Geometry check sheet. Reference: the model listing, model coordinates, mm. Give positions to 0.01 mm unless a question says otherwise; leave off trailing zeros. Write each loop counter-clockwise with the first axis right and the second up, starting at its lowest first coordinate (ties: lowest second). Pieces come first, ordered by that corner, then holes.
(1) Cross-section at C-C (z = 0.85). Record the boundary of the cut face in (x, y) (1 decimal), and give its area (3 significant figures).
(2) Cross-section at B-B (y = 733.5). Record the boundary of the cut face in (x, z) (3 decimals), and give its area (3 significant figures).
(3) Cross-section at D-D (y = 767.5). Record the boundary of the cut face in (x, z) (3 decimals), and give its area (3 significant figures).
(4) Cross-section at A-A (x = -59). Record the boundary of the cut face in (y, z) (3 decimals).
(5) Thickness scan on line 1 along Y through (x, z) = (-29, 2.6); line 2 along Y through (x, z) = (-38, 2.15); line 3 along Y through (x, z) = (-48, 0.6). Record the ranges inside material, lowest first.
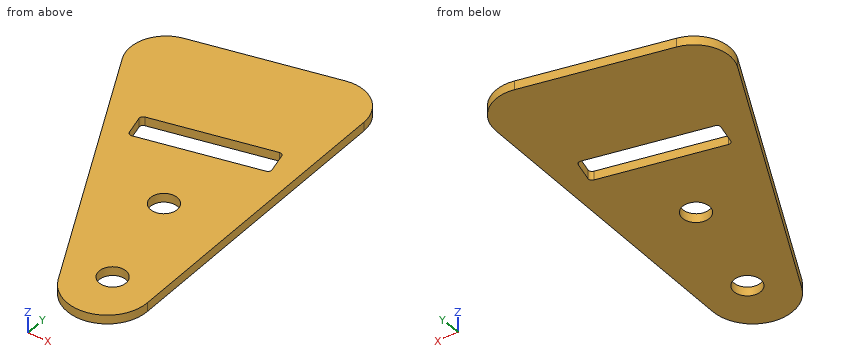
```python
from build123d import *

# Parameters (mm, degrees)
SKETCH1_R           = 4.7625
BOSS_EXTRUDE1_DEPTH = 3.175
FILLET1_R           = 1.27


with BuildPart() as part:
    # Sketch1 → Boss-Extrude1 (new body)
    with BuildSketch(Plane.XY):
        with BuildLine():
            Line((-85.640420597, 747.8061934), (-39.363598028, 654.043532069))
            ThreePointArc((-39.363598028, 654.043532069), (-23.3459714, 646.472574481), (-12.333293773, 660.350783769))
            Line((-12.333293773, 660.350783769), (-12.333293773, 764.911679744))
            ThreePointArc((-12.333293773, 764.911679744), (-17.139019283, 774.860068069), (-27.919188304, 777.279444811))
            Line((-27.919188304, 777.279444811), (-77.137872176, 765.794756196))
            ThreePointArc((-77.137872176, 765.794756196), (-85.733975533, 758.854119696), (-85.640420597, 747.8061934))
        make_face()
        with Locations((-35.934636682, 700.422451369)):
            Circle(SKETCH1_R, mode=Mode.SUBTRACT)
        with Locations((-27.475367191, 664.169477971)):
            Circle(SKETCH1_R, mode=Mode.SUBTRACT)
        Polygon((-63.350014613, 720.107666072), (-20.062836878, 730.208296933), (-22.227257777, 739.484120734), (-65.514435511, 729.383489872), align=None, mode=Mode.SUBTRACT)
    extrude(amount=BOSS_EXTRUDE1_DEPTH)

    # Fillet1
    fillet1_edges = [part.edges().sort_by_distance(p)[0] for p in [
        (-20.062836878, 730.208296933, 1.5875),
        (-22.227257777, 739.484120734, 1.5875),
        (-65.514435511, 729.383489872, 1.5875),
        (-63.350014613, 720.107666072, 1.5875),
    ]]
    fillet(fillet1_edges, radius=FILLET1_R)


solid = part.part
```
Reply:
1. outline: (-85.6, 747.8) - (-39.4, 654) arc R14.3 ccw to (-12.3, 660.4) - (-12.3, 764.9) arc R12.7 ccw to (-27.9, 777.3) - (-77.1, 765.8) arc R12.7 ccw to start; hole (-65.2, 728.1) - (-63.6, 721.3) arc R1.3 ccw to (-62.1, 720.4) - (-21.3, 729.9) arc R1.3 ccw to (-20.4, 731.4) - (-21.9, 738.2) arc R1.3 ccw to (-23.5, 739.2) - (-64.3, 729.7) arc R1.3 ccw to start; hole circle Ø9.5 at (-35.9, 700.4); hole circle Ø9.5 at (-27.5, 664.2)
1. area: 6,020 mm2
2. outline: (-78.58, 0) - (-47.873, 0) - (-47.873, 3.175) - (-78.58, 3.175) - close; (-20.831, 0) - (-12.333, 0) - (-12.333, 3.175) - (-20.831, 3.175) - close
2. area: 124 mm2
3. outline: (-69.83, 0) - (-12.6, 0) - (-12.6, 3.175) - (-69.83, 3.175) - close
3. area: 182 mm2
4. outline: (693.829, 0) - (721.123, 0) - (721.123, 3.175) - (693.829, 3.175) - close; (730.904, 0) - (770.027, 0) - (770.027, 3.175) - (730.904, 3.175) - close
5. line 1: y = 646.31 to 659.66, 668.68 to 728.12, 737.9 to 777.03
5. line 2: y = 651.82 to 696.13, 704.71 to 726.02, 735.8 to 774.93
5. line 3: y = 671.54 to 723.69, 733.47 to 772.59
